Verification items for the finished model (mm, model axes). Face numbers are marked on the shaded views. A direction names the side the tool comes from. Coordinates: 2 decimals unless noted, no trailing zeros. Write each loop counter-clockwise with the first axis right and the second up, starting at its lowest first coordinate (ties: lowest second). Pieces come first, ordered by that corner, then holes. Notation, with made-up numbers: (46.5, 77) - (52.5, 77) arc R12 cw to (52.5, 81) - close; hole circle Ø8 at (26, -30). An arc over 180 degrees is marked (long way). Use CSV: the item, a comma, the result in double quotes. Start each with the question number.
```python
from build123d import *

# Parameters (mm, degrees)
SKETCH_1_R               = 2.5
EXTRUDE_1_DEPTH          = 10.4
SKETCH_2_R               = 3.25
EXTRUDE_2_DEPTH          = 15
CUT_EXTRUDE_1_DEPTH      = 16.68837149
CUT_EXTRUDE_1_DEPTH_BACK = 16.68837149
FILLET_1_R               = 0.5
CUT_EXTRUDE_2_DEPTH      = 16.68837149
CUT_EXTRUDE_2_DEPTH_BACK = 16.68837149
SKETCH_5_R               = 1
SKETCH_6_R               = 2
EXTRUDE_3_DEPTH          = 5


with BuildPart() as part:
    # Эскиз1 → Бобышка-Вытянуть1 (new body)
    with BuildSketch(Plane.XY):
        Circle(SKETCH_1_R)
    extrude(amount=EXTRUDE_1_DEPTH)

    # Эскиз2 → Бобышка-Вытянуть2 (add)
    with BuildSketch(Plane(origin=(0, 0, 0), x_dir=(-1, 0, 0), z_dir=(0, 0, -1))):
        Circle(SKETCH_2_R)
    extrude(amount=EXTRUDE_2_DEPTH)

    # Эскиз4 → Вырез-Вытянуть1 (cut, two sides: drawn at the far end of the back side and taken through both)
    with BuildSketch(Plane(origin=(0, 0, 0), x_dir=(1, 0, 0), z_dir=(0, 1, 0)).offset(-CUT_EXTRUDE_1_DEPTH_BACK)):
        Polygon((-0.45, -10.4), (-0.55, -7.8), (-2.5, -7.8), (-2.5, -10.4), align=None)
        Polygon((0.45, -10.4), (0.55, -7.8), (2.5, -7.8), (2.5, -10.4), align=None)
    extrude(amount=CUT_EXTRUDE_1_DEPTH + CUT_EXTRUDE_1_DEPTH_BACK, mode=Mode.SUBTRACT)

    # Скругление1
    fillet_1_edges = [part.edges().sort_by_distance(p)[0] for p in [
        (0.55, 0, 7.8),
        (-0.55, 0, 7.8),
    ]]
    fillet(fillet_1_edges, radius=FILLET_1_R)

    # Эскиз5 → Вырез-Вытянуть2 (cut, two sides: drawn at the far end of the back side and taken through both)
    with BuildSketch(Plane(origin=(0, 0, 0), x_dir=(1, 0, 0), z_dir=(0, 1, 0)).offset(-CUT_EXTRUDE_2_DEPTH_BACK)):
        with Locations(Location((0, 3, 0), (0, 0, 270))):
            Circle(SKETCH_5_R)
    extrude(amount=CUT_EXTRUDE_2_DEPTH + CUT_EXTRUDE_2_DEPTH_BACK, mode=Mode.SUBTRACT)

    # Эскиз6 → Бобышка-Вытянуть3 (add)
    with BuildSketch(Plane(origin=(0, 0, -15), x_dir=(-1, 0, 0), z_dir=(0, 0, -1))):
        Circle(SKETCH_6_R)
    extrude(amount=EXTRUDE_3_DEPTH)


solid = part.part
```
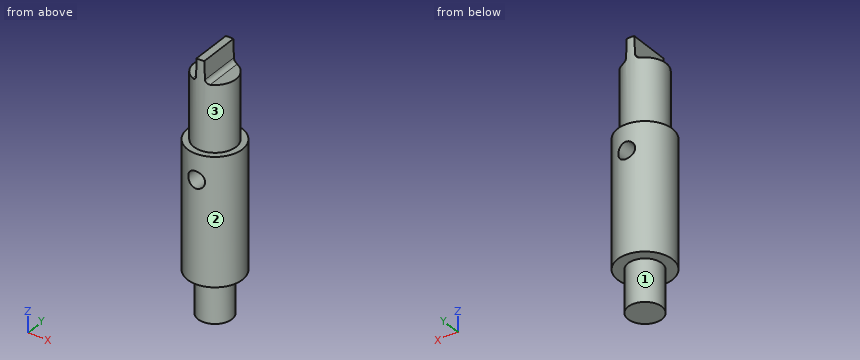
Q1. Cross-section at C-C (z = 3.5). Record the cut outline in (x, y).
Q2. Cross-section at D-D (z = -14.5). Record the cut outline in (x, y), plus the area to 3 significant figures.
Q3. Cross-section at B-B (z = -3). Record the cut outline in (x, y), plus the area to 3 significant figures.
Q4. Cross-section at A-A (y = 0). Record the cut outline in (x, z), plus the area to 3 significant figures.
Q5. Scan lines: line 1 along Z through (x, y) = (0, 1.75); line 2 along X through (y, z) = (-0.25, -3); line 3 along Y through (x, z) = (0, 3.5). Record each from-to range of solid material in increasing order. Write a range as from..to.
Q6. Gauge pin test, flat end, axial feed: pin 1 (1.5 mm diameter, centred on x = -2, y = -1, fed in from +Z). Record the tip position at first contact, or that the pin passes through.
Q7. Tool access check on the marked faces 1, 2 and 3. Record the directions out of +Z, -Z, +X, -X, +Y, -Y that give a thin tool (end or side, any length) a straight path to the whole face; none if there is none.
Reply:
1,outline,"circle Ø5 at (0, 0)"
2,outline,"circle Ø6.5 at (0, 0)"
2,area,"33.2 mm^2"
3,outline,"(-1, -3.09) - (-1, 3.09) arc R3.25 ccw to start; (1, -3.09) arc R3.25 ccw to (1, 3.09) - close"
3,area,"20.4 mm^2"
4,outline,"(-3.25, -15) - (-2, -15) - (-2, -20) - (2, -20) - (2, -15) - (3.25, -15) - (3.25, 0) - (2.5, 0) - (2.5, 7.8) - (1.03, 7.8) arc R0.5 cw to (0.53, 8.28) - (0.45, 10.4) - (-0.45, 10.4) - (-0.53, 8.28) arc R0.5 cw to (-1.03, 7.8) - (-2.5, 7.8) - (-2.5, 0) - (-3.25, 0) - close; hole circle Ø2 at (0, -3)"
4,area,"156 mm^2"
5,line 1,"-20..-4, -2..10.4"
5,line 2,"-3.24..-1, 1..3.24"
5,line 3,"-2.5..2.5"
6,pin 1,"z = 7.8"
7,face 1,"-Z"
7,face 2,"+Z, -Z"
7,face 3,"+Z"
